from build123d import *

# Parameters (mm, degrees)
BOSS_EXTRUDE1_DEPTH = 19.05
SKETCH2_R           = 6.35
CUT_EXTRUDE1_DEPTH  = 21.43
SKETCH3_R           = 4.765
CUT_EXTRUDE2_DEPTH  = 46.1


with BuildPart() as part:
    # Sketch1 → Boss-Extrude1 (new, symmetric)
    with BuildSketch(Plane.XY):
        with BuildLine():
            Line((-3.494114249, 0), (-44.59, 0))
            ThreePointArc((-44.59, 0), (-51.328727625, 2.791272375), (-54.12, 9.53))
            Line((-54.12, 9.53), (-54.12, 85.72))
            ThreePointArc((-54.12, 85.72), (-51.328727625, 92.458727625), (-44.59, 95.25))
            Line((-44.59, 95.25), (9.39, 95.25))
            Line((9.39, 95.25), (9.39, 88.9))
            Line((9.39, 88.9), (-44.59, 88.9))
            ThreePointArc((-44.59, 88.9), (-46.838599564, 87.968599564), (-47.77, 85.72))
            Line((-47.77, 85.72), (-47.77, 9.53))
            ThreePointArc((-47.77, 9.53), (-46.838599564, 7.281400436), (-44.59, 6.35))
            Line((-44.59, 6.35), (-3.494114249, 6.35))
            ThreePointArc((-3.494114249, 6.35), (-2.382548783, 6.545998982), (-1.405054517, 7.11035556))
            Line((-1.405054517, 7.11035556), (30.459242619, 33.847675535))
            Line((30.459242619, 33.847675535), (34.54094394, 28.983293321))
            Line((34.54094394, 28.983293321), (2.676646804, 2.245973346))
            ThreePointArc((2.676646804, 2.245973346), (-0.210720873, 0.57895084), (-3.494114249, 0))
        make_face()
    extrude(amount=BOSS_EXTRUDE1_DEPTH, both=True)

    # Sketch2 → Cut-Extrude1 (cut)
    with BuildSketch(Plane(origin=(0, 95.25, 0), x_dir=(1, 0, 0), z_dir=(0, 1, 0))):
        with Locations(Location((-9.65, 0, 0), (0, 0, 270))):
            Circle(SKETCH2_R)
    extrude(amount=-CUT_EXTRUDE1_DEPTH, mode=Mode.SUBTRACT)

    # Sketch3 → Cut-Extrude2 (cut)
    with BuildSketch(Plane(origin=(-4.081701322, 4.864382214, 0), x_dir=(0.7660444431189815, 0.6427876096865353, 0), z_dir=(-0.6427876096865353, 0.7660444431189815, 0))):
        with Locations(Location((25.29, 0, 0), (0, 0, 180))):
            Circle(SKETCH3_R)
    extrude(amount=-CUT_EXTRUDE2_DEPTH, mode=Mode.SUBTRACT)


solid = part.part
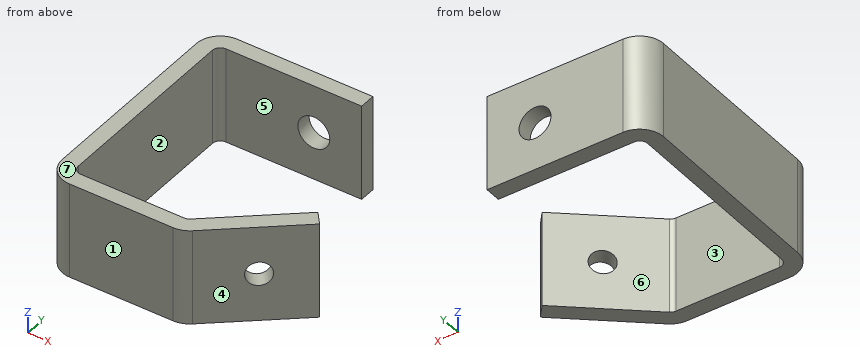
Check sheet for the modelled part. Datum: model origin and axes. Units: mm. Face numbers are marked on the shaded views. A direction names the side the tool comes from. Give positions to 0.01 mm unless a question says otherwise; leave off trailing zeros. Loops run counter-clockwise (first coordinate to the right, second up) from the corner with the lowest first, then second, coordinate; pieces in that order, holes last. Notation, with made-up numbers: M 33,60 L 77,60 A27 ccw 77,76 Z; hole C -31.75,-12 d2. An arc over 180 degrees is marked long. Return JSON: item names as keys, results as strings. Group by question number.
1. Thickness scan on L1, parallel to Y at x = -35, z = 16; L2, parallel to X at y = 61.5, z = -9.5. Record the ranges inside material, lowest first.
2. Cross-section at A-A on x = -33.5. Record the boundary of the cut face in (y, z).
3. Tool access check on the marked faces 5, 6 and 7. Record the directions out of +Z, -Z, +X, -X, +Y, -Y that give a thin tool (end or side, any length) a straight path to the whole face; none if there is none.
4. Cross-section at B-B on x = -9.65. Record the boundary of the cut face in (y, z), plus the area to 3 significant figures.
5. Mould release check, pull along X, two halves, no side actions. Record for the marked faces 1, 2, 3 and 4: released by +X, released by -X, zero draft, split by the parting line, or undercut.
6. Cross-section at C-C on z = 9.5. Record the boundary of the cut face in (x, y), plus the area to 3 significant figures.
7. Cross-section at D-D on z = 0. Record the boundary of the cut face in (x, y).
8. Go/stop test with flat-tipped pins: pin 1 (1 mm diameter, centred on y = 65, z = 13.5, fed in from +X); pin 2 (1 mm diameter, centred on y = 13, z = -13, fed in from +X); pin 3 (1.9 mm diameter, centred on y = 92, z = -8.5, fed in from +X). Record where each tip stops, or that it passes through.
Return value:
{
 "1": {"L1": "0 to 6.35, 88.9 to 95.25", "L2": "-54.12 to -47.77"},
 "2": {"outline": "M 0,-19.05 L 6.35,-19.05 L 6.35,19.05 L 0,19.05 Z; M 88.9,-19.05 L 95.25,-19.05 L 95.25,19.05 L 88.9,19.05 Z"},
 "3": {"face 5": "+Z, -Z, +X", "face 6": "+Z, -Z", "face 7": "+Z, +X, -X, +Y, -Y"},
 "4": {"outline": "M 0,-19.05 L 6.35,-19.05 L 6.35,19.05 L 0,19.05 Z; M 88.9,-19.05 L 95.25,-19.05 L 95.25,-6.35 L 88.9,-6.35 Z; M 88.9,6.35 L 95.25,6.35 L 95.25,19.05 L 88.9,19.05 Z", "area": "403 mm^2"},
 "5": {"face 1": "zero draft", "face 2": "undercut", "face 3": "undercut", "face 4": "released by +X"},
 "6": {"outline": "M -54.12,9.53 A9.53 ccw -44.59,0 L -3.49,0 A9.6 ccw 2.68,2.25 L 34.54,28.98 L 30.46,33.85 L -1.41,7.11 A3.25 cw -3.49,6.35 L -44.59,6.35 A3.18 cw -47.77,9.53 L -47.77,85.72 A3.18 cw -44.59,88.9 L 9.39,88.9 L 9.39,95.25 L -44.59,95.25 A9.53 ccw -54.12,85.72 Z", "area": "1,510 mm^2"},
 "7": {"outline": "M -54.12,9.53 A9.53 ccw -44.59,0 L -3.49,0 A9.6 ccw 2.68,2.25 L 15.72,13.19 L 11.64,18.06 L -1.41,7.11 A3.25 cw -3.49,6.35 L -44.59,6.35 A3.18 cw -47.77,9.53 L -47.77,85.72 A3.18 cw -44.59,88.9 L -16,88.9 L -16,95.25 L -44.59,95.25 A9.53 ccw -54.12,85.72 Z; M -3.3,88.9 L 9.39,88.9 L 9.39,95.25 L -3.3,95.25 Z; M 18.94,24.18 L 23.02,19.32 L 34.54,28.98 L 30.46,33.85 Z"},
 "8": {"pin 1": "x = -47.77", "pin 2": "x = 16.09", "pin 3": "x = 9.39"}
}
